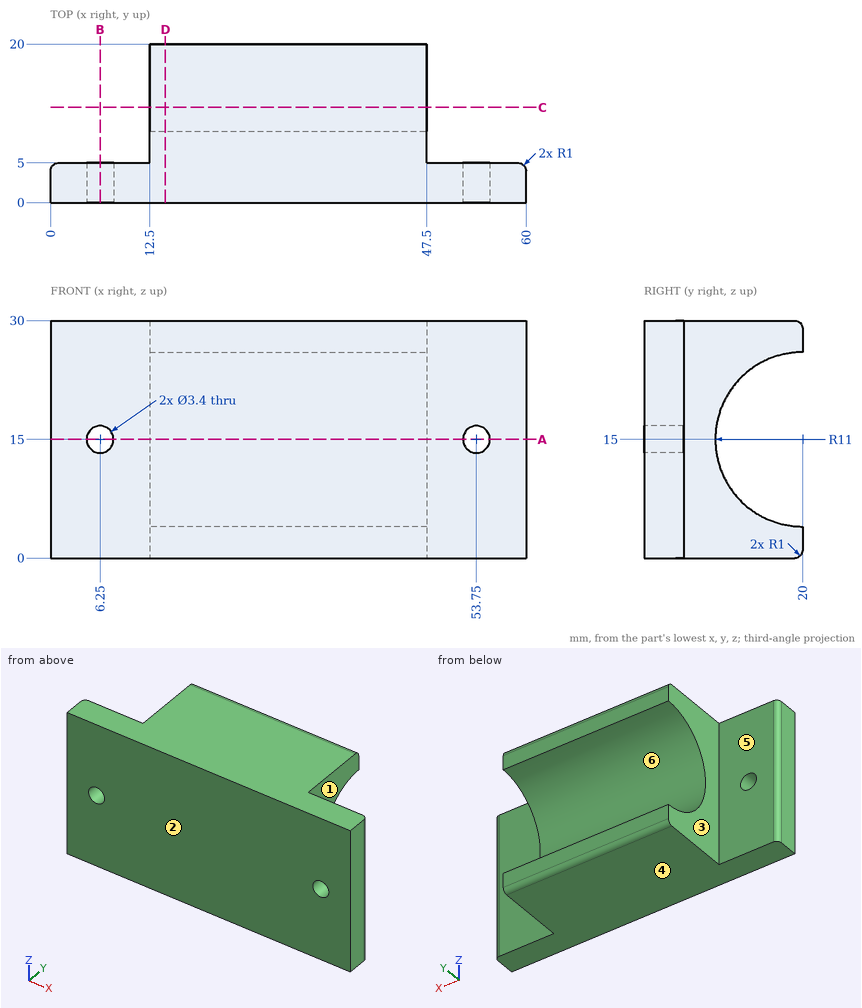
Input: dimensioned drawing with shaded views. Units: mm. Origin: part minimum x, y, z. A direction names the side the tool comes from. Round coordinates to 2 decimals unless told otherwise and drop trailing zeros. Order: outer loops, then holes, each group sorted by start corner. A loop starts at its lowest first (then second) coordinate and runs counter-clockwise, first axis right, second up.
1. Material intervals for line 1 (X direction, y = 1.15, z = 15); line 2 (Z direction, x = 53.75, y = 2.65); line 3 (Y direction, x = 7.5, z = 8.75), sorted ascending.
The answers:
line 1: x = 0 to 4.55, 7.95 to 52.05, 55.45 to 60
line 2: z = 0 to 13.3, 16.7 to 30
line 3: y = 0 to 5
2. Set-up query: the marked faces 1, 2 and 3. Return all of +Z, -Z, +X, -X, +Y, -Y with unobstructed straight access to the full face (end or side cutting, diameter ignored); none if empty.
The answers:
face 1: +Z, -Z, +X, +Y
face 2: +Z, -Z, +X, -X, -Y
face 3: +Z, -Z, -X, +Y
3. Cut plane A-A, the plane z = 15. Output: boundary loops of the cut face in (x, y).
The answers:
outline: (0, 0) - (4.55, 0) - (4.55, 5) - (1, 5) arc R1 ccw to (0, 4) - close; (7.95, 0) - (52.05, 0) - (52.05, 5) - (47.5, 5) - (47.5, 9) - (12.5, 9) - (12.5, 5) - (7.95, 5) - close; (55.45, 0) - (60, 0) - (60, 4) arc R1 ccw to (59, 5) - (55.45, 5) - close
4. Cut plane D-D, the plane x = 14.5. Output: boundary loops of the cut face in (y, z), then the cut area to 3 significant figures.
The answers:
outline: (0, 0) - (19, 0) arc R1 ccw to (20, 1) - (20, 4) arc R11 cw to (20, 26) - (20, 29) arc R1 ccw to (19, 30) - (0, 30) - close
area: 410 mm2
5. Mould query, pull axis Z, two halves, no side actions, for the marked faces 4, 5 and 6. Classes: released by +Z, released by -Z, zero draft, split by the parting line, or undercut.
The answers:
face 4: released by -Z
face 5: zero draft
face 6: undercut
6. Cut plane B-B, the plane x = 6.25. Output: boundary loops of the cut face in (y, z).
The answers:
outline: (0, 0) - (5, 0) - (5, 13.3) - (0, 13.3) - close; (0, 16.7) - (5, 16.7) - (5, 30) - (0, 30) - close
7. Cut plane C-C, the plane y = 12. Output: boundary loops of the cut face in (x, z).
The answers:
outline: (12.5, 0) - (47.5, 0) - (47.5, 7.45) - (12.5, 7.45) - close; (12.5, 22.55) - (47.5, 22.55) - (47.5, 30) - (12.5, 30) - close
8. Pin query (flat end, axial travel): P1, Ø1.5, axis at y = 9, z = 14, coming from the +X side; P2, Ø9, axis at x = 5.5, z = 9.5, coming from the +Y side; P3, Ø3, axis at y = 15.5, z = 5.5, coming from the -X side. Return the tip coordinate at first contact, or that it passes through.
The answers:
P1: stops at x = 47.5
P2: stops at y = 5
P3: stops at x = 12.5
